Geometry check sheet. Reference: the model listing, model coordinates, mm. Face numbers are marked on the shaded views. A direction names the side the tool comes from. Coordinates: 2 decimals unless noted, no trailing zeros. Write each loop counter-clockwise with the first axis right and the second up, starting at its lowest first coordinate (ties: lowest second). Pieces come first, ordered by that corner, then holes. Notation, with made-up numbers: (30, 26.5) -> (49, 26.5) arc R37 ccw to (49, 63.5) -> close; hole circle Ø3 at (51.25, 81.5). An arc over 180 degrees is marked (long way). Answer in a Markdown table with one row per item. Add a question column.
Q1. Tool access check on the marked faces 4 and 5. Record the directions out of +Z, -Z, +X, -X, +Y, -Y that give a thin tool (end or side, any length) a straight path to the whole face; none if there is none.
Q2. Gauge pin test, flat ends, axial feed: P1, Ø8, axis at x = -4, z = 3, coming from the +Y side; P2, Ø2, axis at x = 2, y = 1.5, coming from the +Z side (3 decimals); P3, Ø3, axis at y = 10, z = 19.5, coming from the -X side; P4, Ø1.5, axis at x = -6, z = 19.5, coming from the +Y side. Record the tip position at first contact, or that the pin passes through.
Q3. Release check for a two-part mould opening along Y. For the marked faces 1, 2 and 3 record: pulls with the +Y half, pulls with the -Y half, needs draft (parallel to the pull), parting line crosses it, or undercut.
Q4. Section check D-D, the plane z = 12. Record the boundary of the cut face in (x, y) (3 decimals), and give its area (3 significant figures).
Q5. Thickness scan on line 1 (Y direction, x = 0, z = 15.5) (3 decimals); line 2 (Z direction, x = -11, y = 4.25); line 3 (Z direction, x = 4.25, y = 1) (3 decimals). Record the ranges inside material, lowest first.
Q6. Section check B-B, the plane x = 0. Record the boundary of the cut face in (y, z) (3 decimals).
Q7. Section check A-A, the plane y = 0. Record the boundary of the cut face in (x, z) (3 decimals), and give its area (3 significant figures).
```python
from build123d import *

# Parameters (mm, degrees)
F0_R     = 12.7
F1_DEPTH = 12.7
F2_R     = 9.525
F3_DEPTH = 9.525
F5_DEPTH = 10.16
F6_R     = 5.715
F7_DEPTH = 12.7
F8_R     = 0.381


with BuildPart() as f1:
    # F0 (on Top) → F1 (new body)
    with BuildSketch(Plane.XY):
        Circle(F0_R)
    extrude(amount=F1_DEPTH)

    # F2 (on face) → F3 (join)
    with BuildSketch(Plane.XY.offset(12.7)):
        Circle(F2_R)
    extrude(amount=F3_DEPTH)

    # F4 (on face) → F5 (join)
    with BuildSketch(Plane.XY.offset(22.225)):
        with BuildLine():
            Line((-1.5875, 9.391777), (-1.5875, 6.731))
            Line((-1.5875, 6.731), (1.5875, 6.731))
            Line((1.5875, 6.731), (1.5875, 9.391777))
            ThreePointArc((1.5875, 9.391777), (0, 9.525), (-1.5875, 9.391777))
        make_face()
        with BuildLine():
            Line((-1.5875, 12.319), (-1.5875, 9.391777))
            ThreePointArc((-1.5875, 9.391777), (0, 9.525), (1.5875, 9.391777))
            Line((1.5875, 9.391777), (1.5875, 12.319))
            Line((1.5875, 12.319), (-1.5875, 12.319))
        make_face()
    extrude(amount=-F5_DEPTH)

    # F6 (on face) → F7 (cut)
    with BuildSketch(Plane.XY.offset(22.225)):
        Circle(F6_R)
    extrude(amount=-F7_DEPTH, mode=Mode.SUBTRACT)

    # F8
    f8_edges = [f1.edges().sort_by_distance(p)[0] for p in [
        (1.5875, 12.319, 17.4625),
        (-1.5875, 12.319, 17.4625),
    ]]
    fillet(f8_edges, radius=F8_R)


solid = f1.part
```
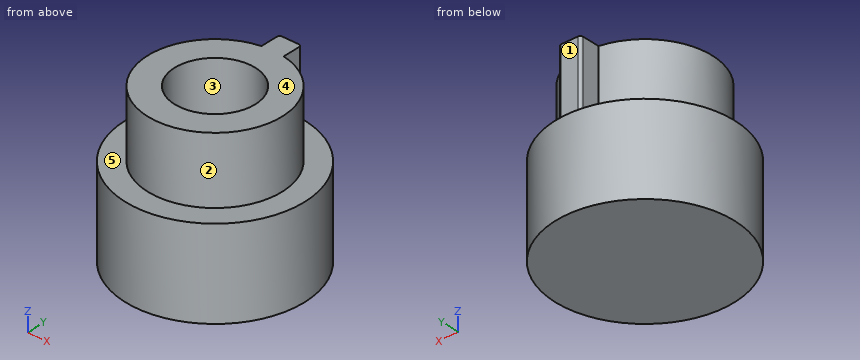
Calculated:
| question | item | result |
|---|---|---|
| 1 | face 4 | +Z, +X, -X, +Y, -Y |
| 1 | face 5 | +Z |
| 2 | P1 | stops at y = 12.7 |
| 2 | P2 | stops at z = 9.525 |
| 2 | P3 | stops at x = -4.3 |
| 2 | P4 | stops at y = 7.95 |
| 3 | face 1 | pulls with the +Y half |
| 3 | face 2 | parting line crosses it |
| 3 | face 3 | undercut |
| 4 | outline | circle Ø25.4 at (0, 0); hole circle Ø11.43 at (0, 0) |
| 4 | area | 404 mm² |
| 5 | line 1 | y = -9.525 to -5.715, 5.715 to 12.319 |
| 5 | line 2 | z = 0 to 12.7 |
| 5 | line 3 | z = 0 to 9.525 |
| 6 | outline | (-12.7, 0) -> (12.7, 0) -> (12.7, 12.7) -> (12.319, 12.7) -> (12.319, 22.225) -> (5.715, 22.225) -> (5.715, 9.525) -> (-5.715, 9.525) -> (-5.715, 22.225) -> (-9.525, 22.225) -> (-9.525, 12.7) -> (-12.7, 12.7) -> close |
| 7 | outline | (-12.7, 0) -> (12.7, 0) -> (12.7, 12.7) -> (9.525, 12.7) -> (9.525, 22.225) -> (5.715, 22.225) -> (5.715, 9.525) -> (-5.715, 9.525) -> (-5.715, 22.225) -> (-9.525, 22.225) -> (-9.525, 12.7) -> (-12.7, 12.7) -> close |
| 7 | area | 359 mm² |
